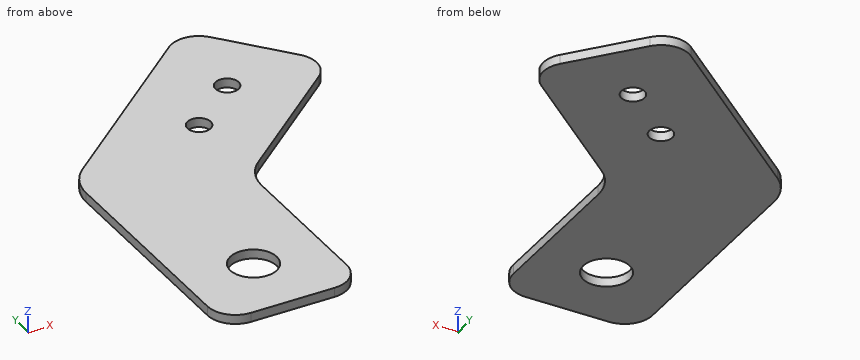
from build123d import *

# Parameters (mm, degrees)
SKETCH1_R          = 5
SKETCH1_R_2        = 2.5
BASE_FLANGE1_DEPTH = 2


# Sheet-metal steps are written as plain solids
with BuildPart() as part:
    # Sketch1 → Base-Flange1 (new body)
    with BuildSketch(Plane.XY):
        with BuildLine():
            Line((-14.238080804, 7.633940989), (-49.730098253, -22.147397762))
            ThreePointArc((-49.730098253, -22.147397762), (-52.365300026, -25.581659576), (-53.302222156, -29.807842194))
            Line((-53.302222156, -29.807842194), (-53.302222156, -48.56164166))
            Line((-53.302222156, -48.56164166), (-53.302222156, -76.139380484))
            ThreePointArc((-53.302222156, -76.139380484), (-51.544862843, -80.382021171), (-47.302222156, -82.139380484))
            Line((-47.302222156, -82.139380484), (-29.302222156, -82.139380484))
            ThreePointArc((-29.302222156, -82.139380484), (-25.059581469, -80.382021171), (-23.302222156, -76.139380484))
            Line((-23.302222156, -76.139380484), (-23.302222156, -48.56164166))
            Line((-23.302222156, -48.56164166), (-23.302222156, -43.797071938))
            ThreePointArc((-23.302222156, -43.797071938), (-22.365300026, -39.570889321), (-19.730098253, -36.136627507))
            Line((-19.730098253, -36.136627507), (5.045547487, -15.347392305))
            ThreePointArc((5.045547487, -15.347392305), (7.165990017, -11.274060103), (5.785088487, -6.894399988))
            Line((5.785088487, -6.894399988), (-5.785088487, 6.894399988))
            ThreePointArc((-5.785088487, 6.894399988), (-9.858420689, 9.014842519), (-14.238080804, 7.633940989))
        make_face()
        with Locations((-38.302222156, -67.139380484)):
            Circle(SKETCH1_R, mode=Mode.SUBTRACT)
        with Locations((-11.490666647, -9.641814145)):
            Circle(SKETCH1_R_2, mode=Mode.SUBTRACT)
        with Locations((-22.981333294, -19.283628291)):
            Circle(SKETCH1_R_2, mode=Mode.SUBTRACT)
    extrude(amount=-BASE_FLANGE1_DEPTH)


solid = part.part
Can you work these out from the model? Positions are in its coordinate system, mm. Coordinates: 2 decimals unless noted, no trailing zeros. Order: outer loops, then holes, each group sorted by start corner. A loop starts at its lowest first (then second) coordinate and runs counter-clockwise, first axis right, second up. Notation, with made-up numbers: M -19.5,85 L -1.5,85 A29 cw -1.5,117 Z; hole C -39,-22.5 d1. An arc over 180 degrees is marked long. Write item = value, one per line.
(1) Suppose I cut it at B-B on x = -41. Please give me the cut outline in (y, z), plus the area to 3 significant figures.
Results are:
outline = M -82.14,-2 L -71.35,-2 L -71.35,0 L -82.14,0 Z; M -62.93,-2 L -14.82,-2 L -14.82,0 L -62.93,0 Z
area = 118 mm2
(2) Suppose I cut it at A-A on z = -0.55. Please give me the cut outline in (x, y).
Results are:
outline = M -53.3,-76.14 A6 ccw -47.3,-82.14 L -29.3,-82.14 A6 ccw -23.3,-76.14 L -23.3,-43.8 A10 cw -19.73,-36.14 L 5.05,-15.35 A6 ccw 5.79,-6.89 L -5.79,6.89 A6 ccw -14.24,7.63 L -49.73,-22.15 A10 ccw -53.3,-29.81 Z; hole C -38.3,-67.14 d10; hole C -22.98,-19.28 d5; hole C -11.49,-9.64 d5
(3) Suppose I cut it at C-C on y = -47. Please give me the cut outline in (x, z).
Results are:
outline = M -53.3,-2 L -23.3,-2 L -23.3,0 L -53.3,0 Z
(4) I need wall thicknesses on line 1 along Y through (x, z) = (-39, -0.45); line 2 along X through (y, z) = (-43.5, -0.1); line 3 along Y through (x, z) = (-40, -0.35). Which ranges of each line are inside material? Lowest first, please. Write a range as [from, to].
Results are:
line_1 = [-82.14, -72.09], [-62.19, -13.14]
line_2 = [-53.3, -23.3]
line_3 = [-82.14, -71.84], [-62.44, -13.98]
(5) Suppose I cut it at D-D on x = -10.5. Please give me the cut outline in (y, z), plus the area to 3 significant figures.
Results are:
outline = M -28.39,-2 L -11.94,-2 L -11.94,0 L -28.39,0 Z; M -7.35,-2 L 9.04,-2 L 9.04,0 L -7.35,0 Z
area = 65.7 mm2
(6) For pin 1 Ø0.6 at (y, z) = (-64.5, -1) entering from +X; pin 2 Ø6.5 at (x, y) = (-11.49, -9.64) entering from -Z, each with a flat end and sliding along its axis, tell me the tip position at first contact or that it passes through.
Results are:
pin_1 = -23.3
pin_2 = -2
